```python
from build123d import *

# Parameters (mm, degrees)
BOSS_EXTRU_1_DEPTH      = 118
BOSS_EXTRU_2_START      = -5
BOSS_EXTRU_2_DEPTH      = 5
CONG_1_R                = 5
ENL_V_MAT_EXTRU_2_DEPTH = 144.326668003
CONG_2_R                = 10
CONG_3_START            = -1
CONG_3_DEPTH            = 119


with BuildPart() as part:
    # Esquisse1 → Boss.-Extru.1 (new body)
    with BuildSketch(Plane.XY):
        with BuildLine():
            Line((-48, 0), (-44.998214382, -0.400877025))
            ThreePointArc((-44.998214382, -0.400877025), (5.956695581, 44.604010781), (43.316094217, -12.194916228))
            Line((43.316094217, -12.194916228), (46.317879834, -12.595793253))
            ThreePointArc((46.317879834, -12.595793253), (6.35380862, 47.5776115), (-48, 0))
        make_face()
    extrude(amount=BOSS_EXTRU_1_DEPTH)

    # Esquisse2 → Boss.-Extru.2 (add)
    with BuildSketch(Plane.XY.offset(118).offset(BOSS_EXTRU_2_START)):
        with BuildLine():
            Line((-58.058892958, 1.511889338), (-47.999984368, 0.038739081))
            ThreePointArc((-47.999984368, 0.038739081), (6.373007198, 47.57504366), (46.317879834, -12.595793253))
            Line((46.317879834, -12.595793253), (43.316094217, -12.194916228))
            Line((43.316094217, -12.194916228), (56.371627647, -14.179393207))
            ThreePointArc((56.371627647, -14.179393207), (7.76570592, 56.450860633), (-58.058892958, 1.511889338))
        make_face()
    extrude(amount=BOSS_EXTRU_2_DEPTH)

    # Congé1
    cong_1_edges = [part.edges().sort_by_distance(p)[0] for p in [
        (6.373007198, 47.57504366, 113),
    ]]
    fillet(cong_1_edges, radius=CONG_1_R)

    # Esquisse4 → Enlèv. mat.-Extru.2 (cut, through all)
    with BuildSketch(Plane(origin=(0, 0, 0), x_dir=(-1, 0, 0), z_dir=(0, 0, -1))):
        with BuildLine():
            ThreePointArc((-43.316094217, -12.194916228), (-44.953602713, -2.042939819), (-44.243666063, 8.215717453))
            Line((-44.243666063, 8.215717453), (-47.362132256, 7.799258183))
            ThreePointArc((-47.362132256, 7.799258183), (-47.93720577, -2.454445548), (-46.317879834, -12.595793253))
            Line((-46.317879834, -12.595793253), (-43.316094217, -12.194916228))
        make_face()
        with BuildLine():
            Line((33.208512529, 30.367658711), (-44.243666063, 8.215717453))
            ThreePointArc((-44.243666063, 8.215717453), (-44.953602713, -2.042939819), (-43.316094217, -12.194916228))
            Line((-43.316094217, -12.194916228), (-46.317879834, -12.595793253))
            ThreePointArc((-46.317879834, -12.595793253), (-47.93720577, -2.454445548), (-47.362132256, 7.799258183))
            Line((-47.362132256, 7.799258183), (-114.354421373, -1.147306612))
            Line((-114.354421373, -1.147306612), (-106.599475071, -56.082579824))
            Line((-106.599475071, -56.082579824), (62.827216074, -36.566785192))
            Line((62.827216074, -36.566785192), (101.490219992, -28.614943218))
            Line((101.490219992, -28.614943218), (87.117247585, 24.85835748))
            Line((87.117247585, 24.85835748), (83.033473236, 40.051658321))
            Line((83.033473236, 40.051658321), (38.369226529, 31.843664105))
            Line((38.369226529, 31.843664105), (36.40632276, 31.28225796))
            ThreePointArc((36.40632276, 31.28225796), (45.008351961, 16.680774975), (48, 0))
            Line((48, 0), (44.998214382, -0.400877025))
            ThreePointArc((44.998214382, -0.400877025), (42.020813074, 16.101281583), (33.208512529, 30.367658711))
        make_face()
        with BuildLine():
            Line((36.186144751, 31.219285292), (33.208512529, 30.367658711))
            ThreePointArc((33.208512529, 30.367658711), (42.020813074, 16.101281583), (44.998214382, -0.400877025))
            Line((44.998214382, -0.400877025), (48, 0))
            ThreePointArc((48, 0), (45.008351961, 16.680774975), (36.40632276, 31.28225796))
            Line((36.40632276, 31.28225796), (36.186144751, 31.219285292))
        make_face()
    extrude(amount=-ENL_V_MAT_EXTRU_2_DEPTH, mode=Mode.SUBTRACT)

    # Congé2
    # the kernel refuses this fillet: 10 mm, written as the material it takes off along each edge
    with BuildSketch(Plane(origin=(-46.806940355, 33.394271389, 157.328464208), x_dir=(0.6968989711094409, 0.7171693133888278, 0), z_dir=(0, 0, -1))) as cong_2_piece_1:
        with BuildLine():
            CenterArc((14.375231745, 9.907615581), CONG_2_R, 196.115404214, 81.678802413)
            Line((4.768186123, 7.131886052), (4.57604521, 7.076371462))
            ThreePointArc((4.57604521, 7.076371462), (2.21782943, 3.677102393), (-0.166263631, 0.111159367))
            Line((-0.166263631, 0.111159367), (-0.027123079, -0.198152312))
            ThreePointArc((-0.027123079, -0.198152312), (7.865692842, -0.735829632), (15.758508762, -0.198152312))
            Line((15.758508762, -0.198152312), (15.731385683, 0))
        make_face()
    extrude(amount=83.656928416, mode=Mode.SUBTRACT)

    # Congé3: read off the stored shape, not the designer's step
    # Congé3 outline → Congé3 (cut)
    with BuildSketch(Plane.XY.offset(CONG_3_START)):
        with BuildLine():
            ThreePointArc((57.403173546, 6.458315401), (55.776215181, 14.490369578), (53.03343531, 22.212936923))
            ThreePointArc((53.03343531, 22.212936923), (52.338794722, 12.890702035), (44.243666063, 8.215717453))
            Line((44.243666063, 8.215717453), (57.403173546, 6.458315401))
        make_face()
    extrude(amount=CONG_3_DEPTH, mode=Mode.SUBTRACT)


solid = part.part
```
Design review of the part built by this model. Coordinates are the model's own, in mm. A direction names the side the tool comes from. Give positions to 0.01 mm unless a question says otherwise; leave off trailing zeros. Order: outer loops, then holes, each group sorted by start corner. A loop starts at its lowest first (then second) coordinate and runs counter-clockwise, first axis right, second up. Notation, with made-up numbers: (-23, 61.25) - (-5, 61.25) arc R20 ccw to (-5, 72.25) - close; hole circle Ø2 at (-31, 4). An arc over 180 degrees is marked (long way). Use a Markdown table: item, result. Add a question column.
(1) Machinability: for faces 1 (the face through (-39.514, 38.632, 115.668)), 2 (the face through (10, 53, 113)), which of the approach directions +Z, -Z, +X, -X, +Y, -Y give a long, thin tool a straight path to every point of the face, cutting with its end or side? Answer none if there is none.
(2) Clearance check with flat-ended pins moving along their axes: P1, Ø8, axis at y = 17.5, z = 57, coming from the +X side; P2, Ø6, axis at x = -23, z = 87, coming from the +Y side; P3, Ø5, axis at x = 29, y = 43, coming from the -Z side. State where each tip first meets the part, or that it passes through.
(3) Add section A-A on z = 104.5. Give the boundary of the cut face in (x, y).
(4) Wall thickness on probe 1 along X at (y, z) = (39, 9); probe 2 along X at (y, z) = (38.5, 110); probe 3 along Y at (x, z) = (1.5, 62.5) (3 decimals): over which ranges is each line inside the solid? List them lowest first. Write a range as [from, to].
Report:
| question | item | result |
|---|---|---|
| 1 | face 1 | +Z, -Z, -X |
| 1 | face 2 | -Z, +Y |
| 2 | P1 | stops at x = 46.06 |
| 2 | P2 | stops at y = 43.63 |
| 2 | P3 | stops at z = 111.43 |
| 3 | outline | (-36.41, 31.28) - (-33.21, 30.37) arc R45 cw to (44.24, 8.22) arc R10 ccw to (47.19, 8.78) arc R48 ccw to start |
| 4 | probe 1 | x = [-27.98, -22.45], [22.45, 27.98] |
| 4 | probe 2 | x = [-29.36, -23.3], [23.3, 29.36] |
| 4 | probe 3 | y = [44.975, 47.977] |
